Job drawing, mm, ordinate dimensions from the low corner. One solid piece. A direction names the side the tool comes from. Coordinates: 2 decimals unless noted, no trailing zeros. Loops run counter-clockwise (first coordinate to the right, second up) from the corner with the lowest first, then second, coordinate; pieces in that order, holes last. Notation, with made-up numbers: (82, 84.5) - (107, 84.5) arc R19 ccw to (107, 95.5) - close; hole circle Ø5 at (19, 67). An arc over 180 degrees is marked (long way). Use a Markdown table: item, result. Add a question column.
1. Drop flat-ended pins along their axis: pin 1 (5 mm diameter, centred on y = 2, z = 9.5, fed in from -X); pin 2 (1.5 mm diameter, centred on x = 5, z = 4.5, fed in from -Y). Give the stop position or say it passes through.
2. Band-saw the part on C-C, the plane z = 5.75. Give the cut face in (x, y), plus the area to 3 significant figures.
3. Wall check: probe 1 along X at (y, z) = (2.5, 5); probe 2 along Z at (x, y) = (13.5, 6); probe 3 along Y at (x, z) = (7, 9.5). Give the ranges that are in metal, low to high. Write a range as [from, to].
4. Band-saw the part on A-A, the plane y = 1. Give the cut face in (x, z), plus the area to 3 significant figures.
5. Pull direction X, two halves, no side cores. Call the marked faces 3, 4 and 5: pulls with the +X half, pulls with the -X half, needs draft (parallel to the pull), parting line crosses it, or undercut.
6. 3-axis set-ups, long thin cutter, end or side, ignore diameter. For the marked faces 1 and 2: which of +Z, -Z, +X, -X, +Y, -Y reach the whole face in a straight line?
7. Band-saw the part on B-B, the plane x = 12.5. Give the cut face in (y, z).
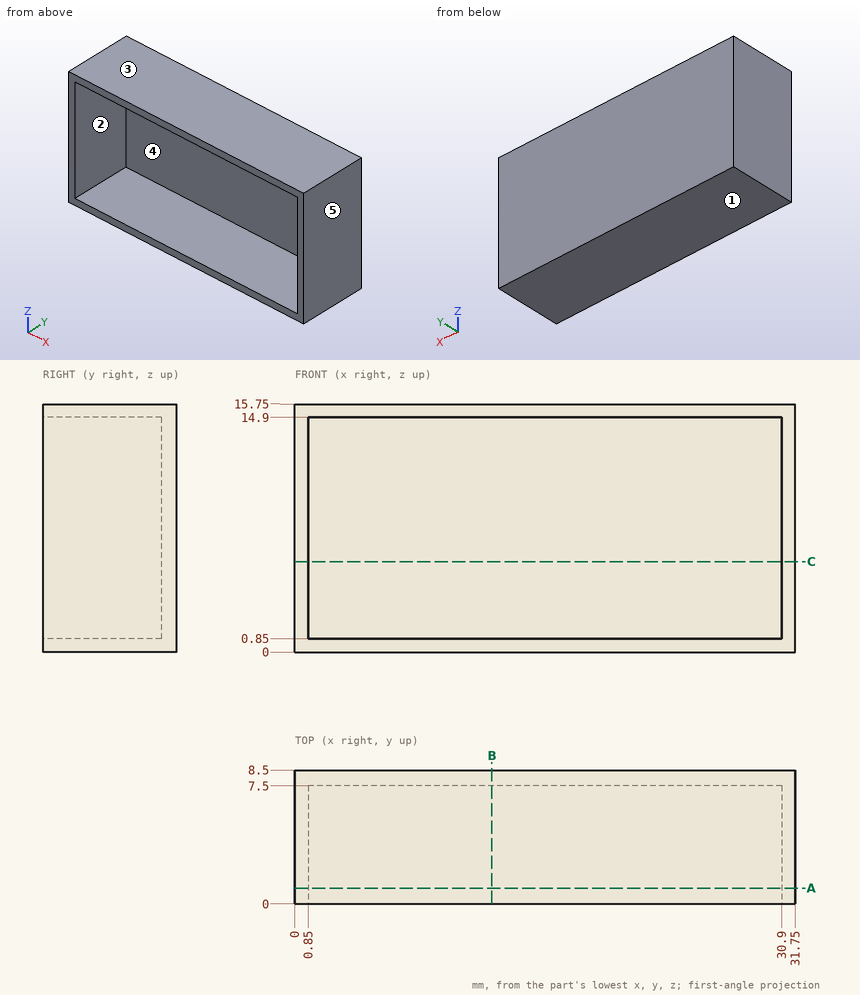
Geometry check:
| question | item | result |
|---|---|---|
| 1 | pin 1 | stops at x = 0 |
| 1 | pin 2 | stops at y = 7.5 |
| 2 | outline | (0, 0) - (0.85, 0) - (0.85, 7.5) - (30.9, 7.5) - (30.9, 0) - (31.75, 0) - (31.75, 8.5) - (0, 8.5) - close |
| 2 | area | 44.5 mm^2 |
| 3 | probe 1 | x = [0, 0.85], [30.9, 31.75] |
| 3 | probe 2 | z = [0, 0.85], [14.9, 15.75] |
| 3 | probe 3 | y = [7.5, 8.5] |
| 4 | outline | (0, 0) - (31.75, 0) - (31.75, 15.75) - (0, 15.75) - close; hole (0.85, 0.85) - (30.9, 0.85) - (30.9, 14.9) - (0.85, 14.9) - close |
| 4 | area | 77.9 mm^2 |
| 5 | face 3 | needs draft |
| 5 | face 4 | undercut |
| 5 | face 5 | pulls with the +X half |
| 6 | face 1 | -Z, +X, -X, +Y, -Y |
| 6 | face 2 | -Y |
| 7 | outline | (0, 0) - (8.5, 0) - (8.5, 15.75) - (0, 15.75) - (0, 14.9) - (7.5, 14.9) - (7.5, 0.85) - (0, 0.85) - close |
